from build123d import *

# Parameters (mm, degrees)
EXTRUDE_1_DEPTH = 50
SKETCH_2_R      = 2.5
EXTRUDE_2_DEPTH = 100
SKETCH_5_R      = 2.5
EXTRUDE_3_DEPTH = 5
SKETCH_6_W      = 8
SKETCH_6_H      = 8
EXTRUDE_4_DEPTH = 8
SKETCH_7_R      = 3
EXTRUDE_5_DEPTH = 60


with BuildPart() as part:
    # 草圖1 → 填料-伸長1 (new body)
    with BuildSketch(Plane(origin=(0, 0, 0), x_dir=(1, 0, 0), z_dir=(0, 1, 0))):
        Polygon((-50, 45), (-50, -45), (-45, -50), (45, -50), (50, -45), (50, 45), (45, 50), (-45, 50), align=None)
    extrude(amount=EXTRUDE_1_DEPTH)

    # 草圖2 → 填料-伸長2 (add)
    with BuildSketch(Plane(origin=(0, 50, 0), x_dir=(1, 0, 0), z_dir=(0, 1, 0))):
        with Locations(Location((40, 0, 0), (0, 0, 90))):
            Circle(SKETCH_2_R)
    extrude(amount=EXTRUDE_2_DEPTH)

    # 草圖4 → 旋轉1 (revolve)
    with BuildSketch(Plane.XY, mode=Mode.PRIVATE) as revolve_1_sk:
        with BuildLine():
            Line((40, 150), (40, 161.880718379))
            add(Edge.make_bspline(
                [(40, 161.880718379), (49.36254318, 162.224748332), (61.644131944, 160.150653719), (70.94600245, 157.886525359)],
                knots=[0, 0, 0, 0, 1, 1, 1, 1], degree=3))
            ThreePointArc((70.94600245, 157.886525359), (73.971530022, 153.523608058), (70, 150))
            Line((70, 150), (40, 150))
        make_face()
    revolve(revolve_1_sk.sketch.rotate(Axis((40, 150, 0), (0, 1, 0)), 90), axis=Axis((40, 150, 0), (0, 1, 0)))

    # 草圖5 → 填料-伸長3 (add)
    with BuildSketch(Plane(origin=(0, 0, -50), x_dir=(-1, 0, 0), z_dir=(0, 0, -1))):
        with Locations(Location((-25, 40, 0), (0, 0, 180))):
            Circle(SKETCH_5_R)
    extrude(amount=EXTRUDE_3_DEPTH)

    # 草圖6 → 填料-伸長4 (add)
    with BuildSketch(Plane(origin=(0, 0, -55), x_dir=(-1, 0, 0), z_dir=(0, 0, -1))):
        with Locations((-25, 40)):
            Rectangle(SKETCH_6_W, SKETCH_6_H)
    extrude(amount=EXTRUDE_4_DEPTH)

    # 草圖7 → 填料-伸長5 (add)
    with BuildSketch(Plane(origin=(0, 44, 0), x_dir=(1, 0, 0), z_dir=(0, 1, 0))):
        with Locations(Location((25, 59, 0), (0, 0, 270))):
            Circle(SKETCH_7_R)
    extrude(amount=EXTRUDE_5_DEPTH)


solid = part.part
For this review, take the finished solid that the model builds, in its own axes (mm). A direction names the side the tool comes from. Round coordinates to 2 decimals unless told otherwise and drop trailing zeros. Write each loop counter-clockwise with the first axis right and the second up, starting at its lowest first coordinate (ties: lowest second). Pieces come first, ordered by that corner, then holes. Notation, with made-up numbers: (83.5, -30.5) - (104.5, -30.5) arc R12 ccw to (104.5, -20.5) - close; hole circle Ø4 at (-26.75, 61.5). An arc over 180 degrees is marked (long way). Write item = value, one per line. Start each with the question number.
1. Consider section D-D on z = -40. State the section outline as (x, y) points, plus the area to 3 significant figures.
2. Draft analysis for pull direction Z (two halves, no side actions). For faces 4 (the face through (27, 42, -55)), 5 (the face through (-1, 25, 50)), 6 (the face through (-47, 25, -48)), state which applies: released by +Z, released by -Z, zero draft, split by the parting line, or undercut.
3. Consider section C-C on x = -24. State the section outline as (y, z) points.
4. Wall thickness on L1, parallel to Y at x = -35, z = 29.5; L2, parallel to X at y = 11.5, z = 26.5; L3, parallel to Y at x = 45.5, z = 30: over which ranges is each line inside the solid? List them lowest first.
5. Consider section A-A on y = 40. State the section outline as (x, z) points.
6. Consider section B-B on y = 84.5. State the section outline as (x, z) points, plus the area to 3 significant figures.
7. For pin 1 Ø5 at (x, z) = (23.5, -57.5) entering from +Y; pin 2 Ø25 at (y, z) = (22.5, -15) entering from +X; pin 3 Ø15 at (x, y) = (1.5, 13) entering from -Z, all flat-tipped, find the tip position at first contact; note any pin that passes through.
8. For faces 1 (the face through (29, 40, -59)), 2 (the face through (42.44, 99.3, 0.54)), 3 (the face through (25, 74, -62)), list the 3-axis set-ups (+Z, -Z, +X, -X, +Y, -Y) from which the entire face can be reached by the end or side of a thin tool; tool diameter is ignored.
Evaluation:
q1.outline = (-50, 0) - (50, 0) - (50, 50) - (-50, 50) - close
q1.area = 5,000 mm2
q2.face_4 = undercut
q2.face_5 = released by +Z
q2.face_6 = released by -Z
q3.outline = (0, -50) - (50, -50) - (50, 50) - (0, 50) - close
q4.L1 = 0 to 50
q4.L2 = -50 to 50
q4.L3 = 0 to 50, 150.03 to 157.99
q5.outline = (-50, -45) - (-45, -50) - (22.5, -50) - (22.5, -55) - (21, -55) - (21, -63) - (29, -63) - (29, -55) - (27.5, -55) - (27.5, -50) - (45, -50) - (50, -45) - (50, 45) - (45, 50) - (-45, 50) - (-50, 45) - close
q6.outline = circle Ø6 at (25, -59); circle Ø5 at (40, 0)
q6.area = 47.9 mm2
q7.pin_1 = 104
q7.pin_2 = 50
q7.pin_3 = -50
q8.face_1 = -Z, +X, +Y, -Y
q8.face_2 = none
q8.face_3 = +Y
